The listing builds one solid part. Answer for the finished solid, in the listing's coordinates (mm). Face numbers are marked on the shaded views. A direction names the side the tool comes from. Give positions to 0.01 mm unless a question says otherwise; leave off trailing zeros. Write each loop counter-clockwise with the first axis right and the second up, starting at its lowest first coordinate (ties: lowest second). Pieces come first, ordered by that corner, then holes. Notation, with made-up numbers: (53, 53.25) -> (82, 53.25) arc R23 cw to (82, 86.25) -> close; hole circle Ø6 at (26.25, 25). An arc over 180 degrees is marked (long way). Put each result on its own line as item: value. Start each with the question number.
1) A cutting plane is placed at D-D (x = 4.25). Write down the section's boundary in (y, z).
2) Find the intervals of material crossed by line 1 along X through (y, z) = (-10, 10.5); line 2 along Y through (x, z) = (3.75, 25); line 3 along Z through (x, y) = (-1, -0.5), in increasing order. Write a range as from..to.
3) Flat-ended cylindrical pins translate along their axes: pin 1 Ø6 at (y, z) = (-6.5, 4.5) entering from +X; pin 2 Ø7 at (x, y) = (5, 2) entering from +Z. Find the tip coordinate at first contact, or state that the pin passes through.
4) For the marked faces 1 and 2, determine the directions among +Z, -Z, +X, -X, +Y, -Y from which every point of the face is accessible in a straight line to the end or side of a thin tool.
5) A cutting plane is placed at B-B (x = 0). Write down the section's boundary in (y, z), then the cut area to 3 significant figures.
6) For a pull along Y with two mould halves and no side action, classify the marked faces 3, 4 and 5 as released by +Y, released by -Y, zero draft, split by the parting line, or undercut.
7) A cutting plane is placed at C-C (y = 1.5). Write down the section's boundary in (x, z), then the cut area to 3 significant figures.
8) A cutting plane is placed at A-A (z = 10.5). Write down the section's boundary in (x, y), then the cut area to 3 significant figures.
from build123d import *

# Parameters (mm, degrees)
SKETCH1_W                    = 19
SKETCH1_H                    = 22
BASE_FLANGE1_DEPTH           = 3
EDGE_FLANGE1_STRIP_W         = 18
EDGE_FLANGE1_STRIP_H         = 3
EDGE_FLANGE1_STRIP_CUT_DEPTH = 19
EDGE_FLANGE1_DEPTH           = 19
SKETCH12_R                   = 2.6
CUT_EXTRUDE1_DEPTH           = 10
SKETCH13_R                   = 2.6
CUT_EXTRUDE2_DEPTH           = 36.146123542
FILLET1_R                    = 7
SKETCH14_R                   = 1.5
CUT_EXTRUDE3_DEPTH           = 36.146123542


# Sheet-metal steps are written as plain solids
with BuildPart() as part:
    # Sketch1 → Base-Flange1 (new body)
    with BuildSketch(Plane.XY):
        Rectangle(SKETCH1_W, SKETCH1_H)
    extrude(amount=-BASE_FLANGE1_DEPTH)

    # Edge-Flange1 strip (across the edge) → Edge-Flange1 strip cut (cut)
    with BuildSketch(Plane(origin=(-9.5, -11, 0), x_dir=(0, 1, 0), z_dir=(1, 0, 0))):
        with Locations((-3, -1.5)):
            Rectangle(EDGE_FLANGE1_STRIP_W, EDGE_FLANGE1_STRIP_H)
    extrude(amount=EDGE_FLANGE1_STRIP_CUT_DEPTH, mode=Mode.SUBTRACT)

    # Edge-Flange1 section (across the edge) → Edge-Flange1 (add)
    with BuildSketch(Plane(origin=(-9.5, -11, 0), x_dir=(0, 1, 0), z_dir=(1, 0, 0))):
        with BuildLine():
            Line((0, 3), (0, 28))
            Line((0, 28), (3, 28))
            Line((3, 28), (3, 3))
            ThreePointArc((3, 3), (3.878679656, 0.878679656), (6, 0))
            Line((6, 0), (6, -3))
            ThreePointArc((6, -3), (1.757359313, -1.242640687), (0, 3))
        make_face()
    extrude(amount=EDGE_FLANGE1_DEPTH)

    # Sketch12 → Cut-Extrude1 (cut)
    with BuildSketch(Plane.XY):
        with Locations((5, 2)):
            Circle(SKETCH12_R)
        with Locations((-5, 2)):
            Circle(SKETCH12_R)
    extrude(amount=-CUT_EXTRUDE1_DEPTH, mode=Mode.SUBTRACT)

    # Sketch13 → Cut-Extrude2 (cut, through all)
    with BuildSketch(Plane(origin=(0, -8, 0), x_dir=(1, 0, 0), z_dir=(0, 1, 0))):
        with Locations(Location((0, -23, 0), (0, 0, 270))):
            Circle(SKETCH13_R)
    extrude(amount=-CUT_EXTRUDE2_DEPTH, mode=Mode.SUBTRACT)

    # Fillet1
    fillet1_edges = [part.edges().sort_by_distance(p)[0] for p in [
        (-9.5, -9.5, 28),
        (9.5, -9.5, 28),
        (-9.5, 11, -1.5),
        (9.5, 11, -1.5),
    ]]
    fillet(fillet1_edges, radius=FILLET1_R)

    # Sketch14 → Cut-Extrude3 (cut, through all)
    with BuildSketch(Plane(origin=(0, -8, 0), x_dir=(1, 0, 0), z_dir=(0, 1, 0))):
        with Locations(Location((0, -10.5, 0), (0, 0, 270))):
            Circle(SKETCH14_R)
    extrude(amount=-CUT_EXTRUDE3_DEPTH, mode=Mode.SUBTRACT)


solid = part.part
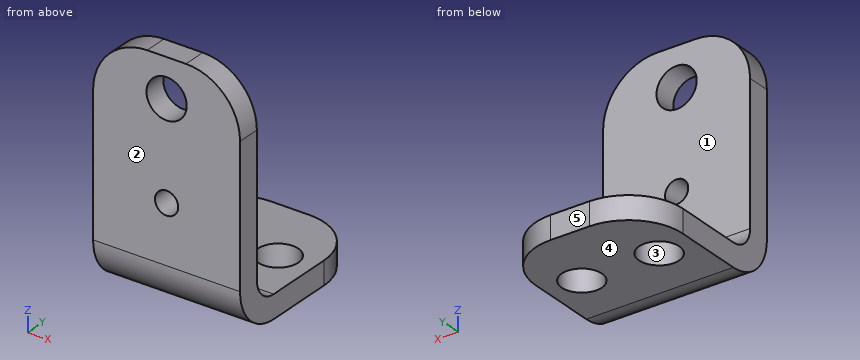
Reply:
1. outline: (-11, 3) arc R6 ccw to (-5, -3) -> (-0.49, -3) -> (-0.49, 0) -> (-5, 0) arc R3 cw to (-8, 3) -> (-8, 27.78) -> (-11, 27.78) -> close; (4.49, -3) -> (10.78, -3) -> (10.78, 0) -> (4.49, 0) -> close
2. line 1: x = -9.5..-1.5, 1.5..9.5
2. line 2: y = -11..-8
2. line 3: z = -3..0
3. pin 1: stops at x = 9.5
3. pin 2: stops at z = 0
4. face 1: +Z, +X, -X, +Y
4. face 2: +Z, -Z, +X, -X, -Y
5. outline: (-11, 3) arc R6 ccw to (-5, -3) -> (11, -3) -> (11, 0) -> (-5, 0) arc R3 cw to (-8, 3) -> (-8, 9) -> (-11, 9) -> close; (-11, 12) -> (-8, 12) -> (-8, 20.4) -> (-11, 20.4) -> close; (-11, 25.6) -> (-8, 25.6) -> (-8, 28) -> (-11, 28) -> close
5. area: 120 mm2
6. face 3: undercut
6. face 4: zero draft
6. face 5: released by +Y
7. outline: (-9.5, -3) -> (-7.55, -3) -> (-7.55, 0) -> (-9.5, 0) -> close; (-2.45, -3) -> (2.45, -3) -> (2.45, 0) -> (-2.45, 0) -> close; (7.55, -3) -> (9.5, -3) -> (9.5, 0) -> (7.55, 0) -> close
7. area: 26.4 mm2
8. outline: (-9.5, -11) -> (-1.5, -11) -> (-1.5, -8) -> (-9.5, -8) -> close; (1.5, -11) -> (9.5, -11) -> (9.5, -8) -> (1.5, -8) -> close
8. area: 48.0 mm2
